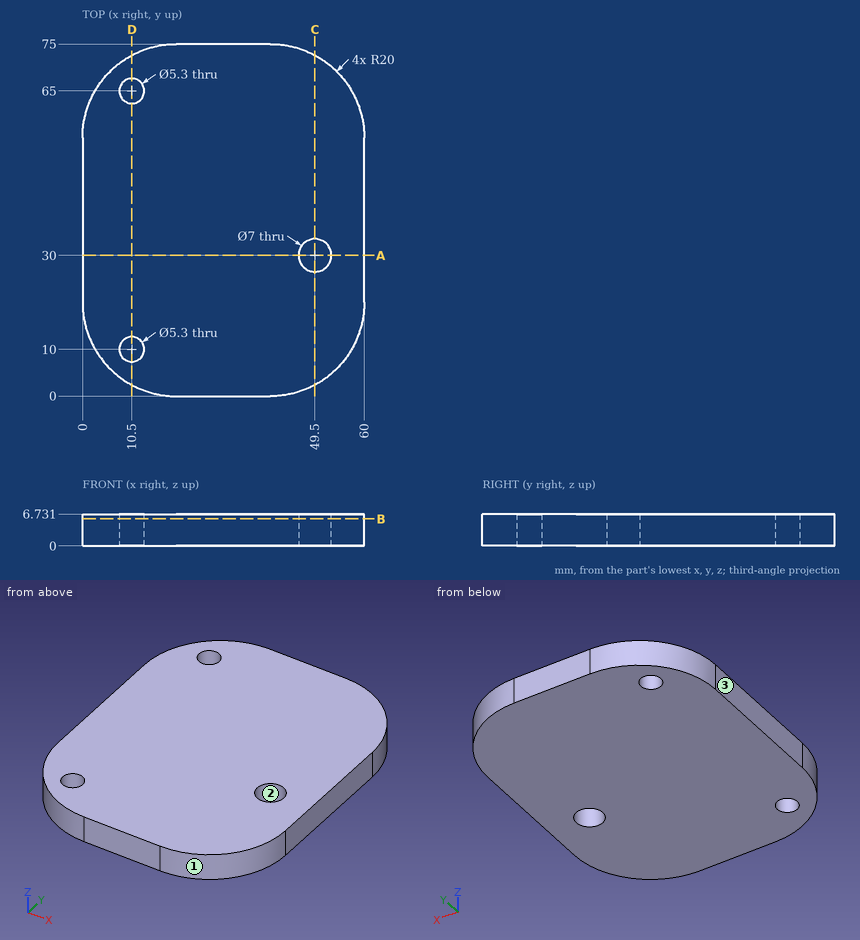
Answer from the drawing. Dimensions are ordinates in mm from the lowest x, y and z of the part. Give positions to 0.01 mm unless a question says otherwise; leave off trailing zeros. Order: outer loops, then holes, each group sorted by start corner. A loop starts at its lowest first (then second) coordinate and runs counter-clockwise, first axis right, second up. Notation, with made-up numbers: (37, 36.25) -> (81, 36.25) arc R26 cw to (81, 66.25) -> close; hole circle Ø5 at (70.5, 52.5). An arc over 180 degrees is marked (long way). One line per item, written item: value.
Item 1: Straight lines are drawn through the part: probe 1 along Y at (x, z) = (10.5, 2); probe 2 along Y at (x, z) = (12, 4.25); probe 3 along Y at (x, z) = (40.5, 2.5). For each, find the intervals that lie inside material, in ascending order.
Answer sheet:
probe 1: 2.4 to 7.35, 12.65 to 62.35, 67.65 to 72.6
probe 2: 1.67 to 7.82, 12.18 to 62.82, 67.18 to 73.33
probe 3: 0.01 to 74.99
Item 2: Find section A-A, the plane y = 30. Give the vertices of the cut face in (x, z).
Answer sheet:
outline: (0, 0) -> (46, 0) -> (46, 6.73) -> (0, 6.73) -> close; (53, 0) -> (60, 0) -> (60, 6.73) -> (53, 6.73) -> close
Item 3: Find section D-D, the plane x = 10.5. Give the vertices of the cut face in (y, z).
Answer sheet:
outline: (2.4, 0) -> (7.35, 0) -> (7.35, 6.73) -> (2.4, 6.73) -> close; (12.65, 0) -> (62.35, 0) -> (62.35, 6.73) -> (12.65, 6.73) -> close; (67.65, 0) -> (72.6, 0) -> (72.6, 6.73) -> (67.65, 6.73) -> close
Item 4: Flat-ended cylindrical pins translate along their axes: P1, Ø6.5, axis at x = 49.5, y = 30, coming from the +Z side; P2, Ø3, axis at x = 15, z = 4, coming from the -Y side. Find the tip coordinate at first contact, or state that the pin passes through.
Answer sheet:
P1: through
P2: y = 0.31
Item 5: Find section B-B, the plane z = 5.75. Give the vertices of the cut face in (x, y).
Answer sheet:
outline: (0, 20) arc R20 ccw to (20, 0) -> (40, 0) arc R20 ccw to (60, 20) -> (60, 55) arc R20 ccw to (40, 75) -> (20, 75) arc R20 ccw to (0, 55) -> close; hole circle Ø5.3 at (10.5, 10); hole circle Ø5.3 at (10.5, 65); hole circle Ø7 at (49.5, 30)
Item 6: Find section C-C, the plane x = 49.5. Give the vertices of the cut face in (y, z).
Answer sheet:
outline: (2.4, 0) -> (26.5, 0) -> (26.5, 6.73) -> (2.4, 6.73) -> close; (33.5, 0) -> (72.6, 0) -> (72.6, 6.73) -> (33.5, 6.73) -> close
Item 7: Determine the mould class of the marked faces 1, 2 and 3 for opening direction X: released by +X, released by -X, zero draft, split by the parting line, or undercut.
Answer sheet:
face 1: released by +X
face 2: undercut
face 3: released by -X
